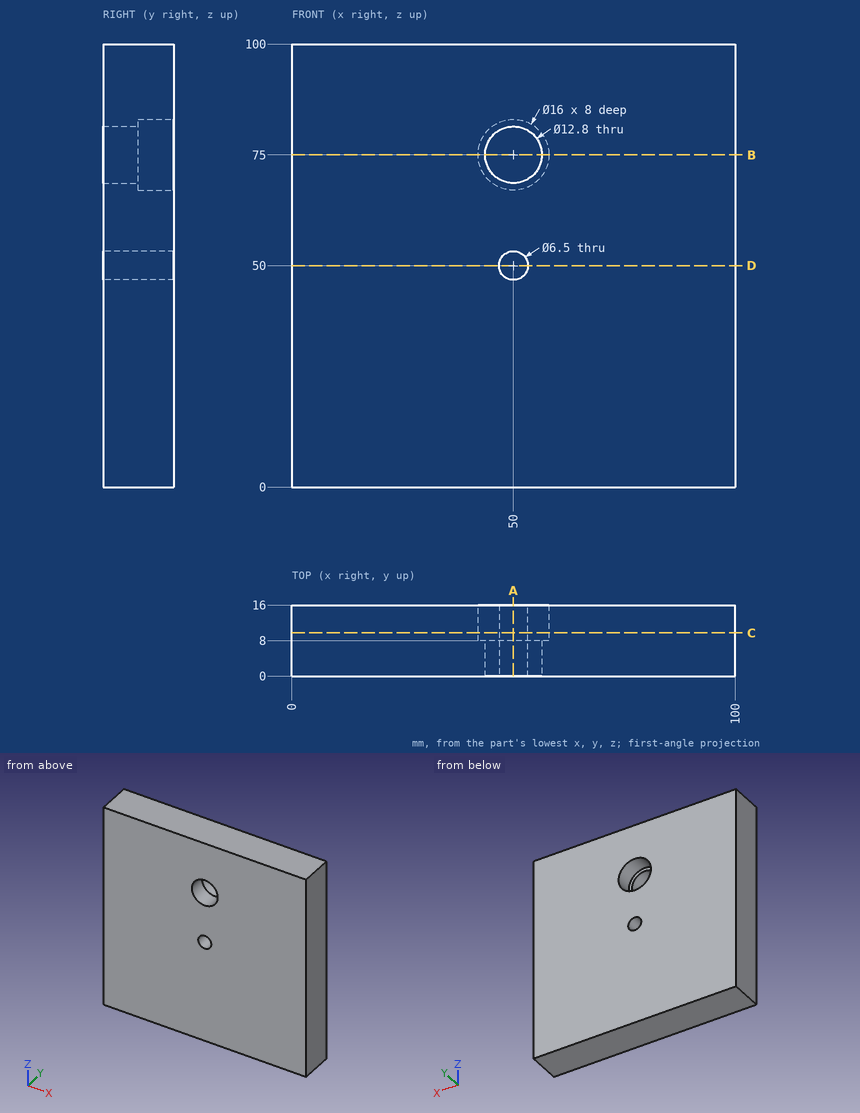
The figure shows three views and two pictorial views of one solid part (mm, origin at its lowest corner). Answer the questions. Coordinates: 2 decimals unless noted, no trailing zeros. Write each loop counter-clockwise with the first axis right and the second up, starting at its lowest first coordinate (ties: lowest second). Pieces come first, ordered by that corner, then holes. Notation, with made-up numbers: (-21, -5.5) -> (1, -5.5) arc R8 cw to (1, 8.5) -> close; hole circle Ø7 at (17.25, 6.5). An arc over 180 degrees is marked (long way). Return JSON: item names as keys, results as strings.
(1) Consider line 1 along Z through (x, y) = (50, 10.75); line 2 along X through (y, z) = (4.5, 75); line 3 along X through (y, z) = (11, 50). Determine where each line is inside the solid, lowest interval first. Write a range as from..to.
Answers below:
{"line 1": "0..46.75, 53.25..67, 83..100", "line 2": "0..43.6, 56.4..100", "line 3": "0..46.75, 53.25..100"}
(2) The part is cut by section B-B on z = 75. Give the vertices of the cut face in (x, y), then the cut area to 3 significant figures.
Answers below:
{"outline": "(0, 0) -> (43.6, 0) -> (43.6, 8) -> (42, 8) -> (42, 16) -> (0, 16) -> close; (56.4, 0) -> (100, 0) -> (100, 16) -> (58, 16) -> (58, 8) -> (56.4, 8) -> close", "area": "1,370 mm^2"}
(3) The part is cut by section D-D on z = 50. Give the vertices of the cut face in (x, y).
Answers below:
{"outline": "(0, 0) -> (46.75, 0) -> (46.75, 16) -> (0, 16) -> close; (53.25, 0) -> (100, 0) -> (100, 16) -> (53.25, 16) -> close"}
(4) The part is cut by section C-C on y = 9.75. Give the vertices of the cut face in (x, z).
Answers below:
{"outline": "(0, 0) -> (100, 0) -> (100, 100) -> (0, 100) -> close; hole circle Ø16 at (50, 75); hole circle Ø6.5 at (50, 50)"}
(5) The part is cut by section A-A on x = 50. Give the vertices of the cut face in (y, z).
Answers below:
{"outline": "(0, 0) -> (16, 0) -> (16, 46.75) -> (0, 46.75) -> close; (0, 53.25) -> (16, 53.25) -> (16, 67) -> (8, 67) -> (8, 68.6) -> (0, 68.6) -> close; (0, 81.4) -> (8, 81.4) -> (8, 83) -> (16, 83) -> (16, 100) -> (0, 100) -> close"}
